Build history of the part. All positions in model axes, mm. A direction names the side the tool comes from. Give positions to 0.01 mm unless a question says otherwise; leave off trailing zeros. Order: outer loops, then holes, each group sorted by start corner. A loop starts at its lowest first (then second) coordinate and runs counter-clockwise, first axis right, second up. Notation, with made-up numbers: (31.5, -24) - (72.5, -24) arc R13 ccw to (72.5, -4) - close; hole circle Ø2 at (-5.75, 42). An arc over 180 degrees is marked (long way). One line per item, written item: value.
```python
from build123d import *

# Parameters (mm, degrees)
F1_DEPTH = 1.05
F2_R     = 1
F4_DEPTH = 12
F5_R     = 2


with BuildPart() as f1:
    # F0 (on Front) → F1 (new body)
    with BuildSketch(Plane.XZ):
        with BuildLine():
            ThreePointArc((-1.102396, 12.451294), (-8.440085, -9.220356), (12.5, 0))
            ThreePointArc((12.5, 0), (9.242496, 8.415834), (1.167797, 12.44533))
            Line((1.167797, 12.44533), (0.567577, 2.434719))
            ThreePointArc((0.567577, 2.434719), (1.958181, 1.554197), (2.5, 0))
            ThreePointArc((2.5, 0), (-1.5644, -1.950039), (-0.542121, 2.440513))
            Line((-0.542121, 2.440513), (-1.102396, 12.451294))
        make_face()
    extrude(amount=F1_DEPTH)

    # F2
    f2_edges = [f1.edges().sort_by_distance(p)[0] for p in [
        (-1.102396, -0.525, 12.451294),
        (1.167797, -0.525, 12.44533),
        (-0.542121, -0.525, 2.440513),
        (0.567577, -0.525, 2.434719),
    ]]
    fillet(f2_edges, radius=F2_R)

    # F3 (on face) → F4 (join)
    with BuildSketch(Plane.XZ.offset(1.05)):
        with BuildLine():
            ThreePointArc((0.860766, 7.324596), (5.510843, 4.901146), (7.375, 0))
            ThreePointArc((7.375, 0), (-4.918049, -5.495764), (-0.815757, 7.329745))
            Line((-0.815757, 7.329745), (-0.891291, 8.679356))
            ThreePointArc((-0.891291, 8.679356), (-5.845901, -6.476965), (8.725, 0))
            ThreePointArc((8.725, 0), (6.493911, 5.82707), (0.941676, 8.674034))
            Line((0.941676, 8.674034), (0.860766, 7.324596))
        make_face()
    extrude(amount=F4_DEPTH)

    # F5
    f5_edges = [f1.edges().sort_by_distance(p)[0] for p in [
        (-0.853524, -13.05, 8.004551),
        (0.901221, -13.05, 7.999315),
    ]]
    fillet(f5_edges, radius=F5_R)


solid = f1.part
```
(1) Drill centre lines: line 1 (X direction, y = -9.25, z = 0) (3 decimals); line 2 (Y direction, x = -8.5, z = 5); line 3 (Z direction, x = 3.5, y = -2). Where is each one in solid material? Low to high.
Completed:
line 1: -8.725 to -7.375, 7.375 to 8.725
line 2: -1.05 to 0
line 3: -7.99 to -6.49, 6.49 to 7.99
(2) Pin check, flat tips, straight feed: P1, Ø4, axis at x = -1.5, y = -7, coming from the +Z side; P2, Ø1.5, axis at x = -6, y = -9, coming from the -Z side; P3, Ø3, axis at y = -10.5, z = -5.5, coming from the -X side. Stop position of each tip, or through.
Completed:
P1: z = 8.68
P2: z = -6.97
P3: x = -7.75
(3) Slice it at B-B, the plane y = -6.5. Give the cut face in (x, z) (3 decimals), and give its area (3 significant figures).
Completed:
outline: (-0.891, 8.679) arc R8.725 ccw (long way) to (0.942, 8.674) - (0.861, 7.325) arc R7.375 cw (long way) to (-0.816, 7.33) - close
area: 65.9 mm²
(4) 3-axis set-ups, long thin cutter, end or side, ignore diameter. For faces 1 (the face through (0, -1.05, -3)), 2 (the face through (1.47, -12.45, 7.95)), 3 (the face through (-1.43, -0.53, 12.11)), 4 (the face through (0.736, -0.532, 2.621)): which of +Z, -Z, +X, -X, +Y, -Y reach the whole face in a straight line?
Completed:
face 1: -Y
face 2: +Z, -Y
face 3: +Z, +Y, -Y
face 4: +Y, -Y
(5) Slice it at A-A, the plane z = 3.5. Give the cut face in (x, y).
Completed:
outline: (-12, -1.05) - (-7.99, -1.05) - (-7.99, -13.05) - (-6.49, -13.05) - (-6.49, -1.05) - (-0.6, -1.05) - (-0.6, 0) - (-12, 0) - close; (0.63, -1.05) - (6.49, -1.05) - (6.49, -13.05) - (7.99, -13.05) - (7.99, -1.05) - (12, -1.05) - (12, 0) - (0.63, 0) - close
(6) Slice it at D-D, the plane z = -2. Give the cut face in (x, y), and give its area (3 significant figures).
Completed:
outline: (-12.34, -1.05) - (-8.49, -1.05) - (-8.49, -13.05) - (-7.1, -13.05) - (-7.1, -1.05) - (-1.5, -1.05) - (-1.5, 0) - (-12.34, 0) - close; (1.5, -1.05) - (7.1, -1.05) - (7.1, -13.05) - (8.49, -13.05) - (8.49, -1.05) - (12.34, -1.05) - (12.34, 0) - (1.5, 0) - close
area: 56.2 mm²
(7) Pull direction X, two halves, no side cores. Call faces 5 (the face through (-0.72, -0.532, 2.616)), 6 (the face through (0, 0, -3)): +X half, -X half, draft (parallel to the pull), parting line (faces both ways), or undercut.
Completed:
face 5: undercut
face 6: draft
(8) Slice it at C-C, the plane x = 0. Give the cut face in (y, z) (3 decimals).
Completed:
outline: (-13.05, -8.725) - (-1.05, -8.725) - (-1.05, -12.5) - (0, -12.5) - (0, -2.5) - (-1.05, -2.5) - (-1.05, -7.375) - (-13.05, -7.375) - close
